Autodesk Inventor part; units mm, degrees
ref_plane "YZ Plane" through (0, 0, 0) normal (1, 0, 0) x (0, 1, 0)
ref_plane "XZ Plane" through (0, 0, 0) normal (0, 1, 0) x (-1, 0, 0)
ref_plane "XY Plane" through (0, 0, 0) normal (0, 0, 1) x (1, 0, 0)
sketch "Boceto1" plane through (0, 0, 0) normal (0, 0, 1) x (1, 0, 0)
  line L0 (10, 0) -> (-10, 0)
  line L1 (-10, 0) -> (-10, 20)
  line L2 (-10, 20) -> (10, 20)
  line L3 (10, 20) -> (10, 0)
  point P0 (0, 0)
  point P1 (0, 0)
  dimension "d0" = 20
  dimension "d1" = 20
extrude "Extrusión1" add sketch "Boceto1" along normal blind 5
sketch "Boceto2" plane through (0, 0, 0) normal (0, 0, 1) x (1, 0, 0)
  line L0 (-10, 0) -> (10, 0) construction
  line L1 (-10, 0) -> (10, 0)
  line L2 (10, 0) -> (10, 5)
  line L3 (10, 5) -> (-10, 5)
  line L4 (-10, 5) -> (-10, 0)
  point P0 (0, 0)
  dimension "d4" = 5
extrude "Extrusión2" add sketch "Boceto2" along normal blind 20
sketch "Boceto3" plane through (0, 0, 5) normal (0, 0, 1) x (1, 0, 0)
  line L0 (-10, 20) -> (-10, 5) construction
  line L1 (10, 20) -> (-10, 20) construction
  line L2 (10, 5) -> (10, 20) construction
  point P0 (0, 0)
  point P1 (-5, 15)
  point P2 (5, 15)
  dimension "d7" = 5
  dimension "d8" = 5
  dimension "d9" = 5
  dimension "d10" = 5
sketch "Boceto4" plane through (-10, 5, 5) normal (0, 1, 0) x (1, 0, 0)
  line L0 (0, 0) -> (0, -15) construction
  line L1 (20, -15) -> (0, -15) construction
  line L2 (20, 0) -> (20, -15) construction
  point P0 (10, 5)
  point P1 (5, -10)
  point P2 (15, -10)
  dimension "d14" = 5
  dimension "d15" = 5
  dimension "d16" = 5
  dimension "d17" = 5
hole "Agujero1" at (-5, 5, 15) at (5, 5, 15) direction (0, -1, 0) diameter 3.2 end through all counterbore diameter 6.2 counterbore depth 1.5
hole "Agujero2" at (-5, 15, 5) at (5, 15, 5) direction (0, 0, -1) diameter 3.2 end through all counterbore diameter 6.2 counterbore depth 1.5
sketch "Boceto5" plane through (0, 0, 0) normal (1, 0, 0) x (0, 1, 0)
  line L0 (5, 5) -> (5, 20) construction
  line L1 (5, 20) -> (20, 5)
  line L2 (20, 5) -> (5, 5) construction
  line L3 (5, 5) -> (20, 5) construction
  line L4 (5, 20) -> (5, 5)
  line L5 (20, 5) -> (5, 5)
  point P0 (0, 0)
  dimension "d32" = 45
  dimension "d33" = 15
extrude "Extrusión4" add sketch "Boceto5" along normal mid plane 4
sketch "Boceto6" plane through (0, 0, 0) normal (1, 0, 0) x (0, 1, 0)
  line L0 (5, 5) -> (5, 20) construction
  line L1 (5, 10) -> (10, 5)
  line L2 (5, 5) -> (20, 5) construction
  line L3 (5, 5) -> (10, 5)
  line L4 (5, 10) -> (5, 5)
  point P0 (0, 0)
  dimension "d36" = 45
  dimension "d37" = 5
extrude "Extrusión5" add sketch "Boceto6" along normal mid plane 20
chamfer "Chaflán1" distance 1 angle 45 9 edges at (-10, 0, 10) (0, 0, 20) (10, 0, 10) (0, 0, 0) (-10, 10, 0) (10, 10, 0) (0, 20, 0) (-2, 12.5, 12.5) (2, 12.5, 12.5)
fillet "Empalme1" radius 1 4 edges at (-10, 3, 20) (-10, 20, 3) (10, 20, 3) (10, 3, 20)
properties part number "T"
Geometry check sheet. Reference: the model listing, model coordinates, mm. A direction names the side the tool comes from. Coordinates: 2 decimals unless noted, no trailing zeros. Order: outer loops, then holes, each group sorted by start corner. A loop starts at its lowest first (then second) coordinate and runs counter-clockwise, first axis right, second up. Notation, with made-up numbers: (-21.5, 71) -> (20.5, 71) arc R9 cw to (20.5, 76) -> close; hole circle Ø1 at (15, 27.25). An arc over 180 degrees is marked (long way). Use a Markdown table: item, result. Add a question column.
1. Set-up check for faces 5 (the face through (9, 5, 15)), 6 (the face through (0, 10, 0)), 7 (the face through (-6, 7, 8)): record each of +Z, -Z, +X, -X, +Y, -Y from which the full face is reachable in a straight line by a thin tool's end or side.
2. Mould release check, pull along X, two halves, no side actions. Record for faces 1 (the face through (0, 0, 10)), 2 (the face through (4.93, 1.73, 13.4)), 3 (the face through (9.5, 0.5, 10.5)), 4 (the face through (-9.5, 0.5, 10.2)): pulls with the +X half, pulls with the -X half, needs draft (parallel to the pull), parting line crosses it, or undercut.
3. Cross-section at D-D (x = -0.25). Enter the section's corners in (y, z), and give its area (3 significant figures).
4. Cross-section at C-C (z = 2.75). Enter the section's corners in (x, y), and give its area (3 significant figures).
5. Go/stop test with flat-tipped pins: pin 1 Ø4.5 at (x, z) = (-4, 14.5) entering from +Y; pin 2 Ø3 at (y, z) = (11, 16) entering from +X; pin 3 Ø7 at (y, z) = (11.5, 15) entering from +X; pin 4 Ø2.5 at (x, z) = (-5, 15) entering from -Y. Record where each tip stops, or that it passes through.
6. Cross-section at A-A (x = 5). Enter the section's corners in (y, z).
7. Cross-section at B-B (y = 4.5). Enter the section's corners in (x, z).
8. Material ranges on L1, parallel to X at y = 15, z = 2.2; L2, parallel to X at y = 4.2, z = 15; L3, parallel to Z at x = 5, y = 1.7, recorded low to high.
Filled sheet:
| question | item | result |
|---|---|---|
| 1 | face 5 | +Z, +X, +Y |
| 1 | face 6 | -Z, +X, -X, +Y, -Y |
| 1 | face 7 | +Z, -X, +Y |
| 2 | face 1 | needs draft |
| 2 | face 2 | undercut |
| 2 | face 3 | pulls with the +X half |
| 2 | face 4 | pulls with the -X half |
| 3 | outline | (0, 1) -> (1, 0) -> (19, 0) -> (20, 1) -> (20, 5) -> (5, 20) -> (1, 20) -> (0, 19) -> close |
| 3 | area | 286 mm2 |
| 4 | outline | (-10, 1) -> (-9, 0) -> (9, 0) -> (10, 1) -> (10, 19) arc R1 ccw to (9, 20) -> (-9, 20) arc R1 ccw to (-10, 19) -> close; hole circle Ø3.2 at (-5, 15); hole circle Ø3.2 at (5, 15) |
| 4 | area | 382 mm2 |
| 5 | pin 1 | y = 10.12 |
| 5 | pin 2 | x = 1.09 |
| 5 | pin 3 | x = 2 |
| 5 | pin 4 | through |
| 6 | outline | (0, 1) -> (1, 0) -> (13.4, 0) -> (13.4, 3.5) -> (11.9, 3.5) -> (11.9, 5) -> (10, 5) -> (5, 10) -> (5, 11.9) -> (3.5, 11.9) -> (3.5, 13.4) -> (0, 13.4) -> close; (0, 16.6) -> (3.5, 16.6) -> (3.5, 18.1) -> (5, 18.1) -> (5, 20) -> (1, 20) -> (0, 19) -> close; (16.6, 0) -> (19, 0) -> (20, 1) -> (20, 5) -> (18.1, 5) -> (18.1, 3.5) -> (16.6, 3.5) -> close |
| 7 | outline | (-10, 1) -> (-9, 0) -> (9, 0) -> (10, 1) -> (10, 19) arc R1 ccw to (9, 20) -> (-9, 20) arc R1 ccw to (-10, 19) -> close; hole circle Ø6.2 at (-5, 15); hole circle Ø6.2 at (5, 15) |
| 8 | L1 | -10 to -6.6, -3.4 to 3.4, 6.6 to 10 |
| 8 | L2 | -10 to -8.1, -1.9 to 1.9, 8.1 to 10 |
| 8 | L3 | 0 to 13.4, 16.6 to 20 |
